Check sheet for the drawn part. Datum: minimum x, y, z corner. Units: mm. A direction names the side the tool comes from. Give positions to 0.01 mm unless a question says otherwise; leave off trailing zeros. Write each loop counter-clockwise with the first axis right and the second up, starting at its lowest first coordinate (ties: lowest second). Pieces come first, ordered by that corner, then holes. Notation, with made-up numbers: (-32.75, 20.5) - (-13.75, 20.5) arc R13 ccw to (-13.75, 26.5) - close; hole circle Ø5 at (10, 27). An arc over 180 degrees is marked (long way). Return JSON: item names as keys, results as strings. Group by question number.
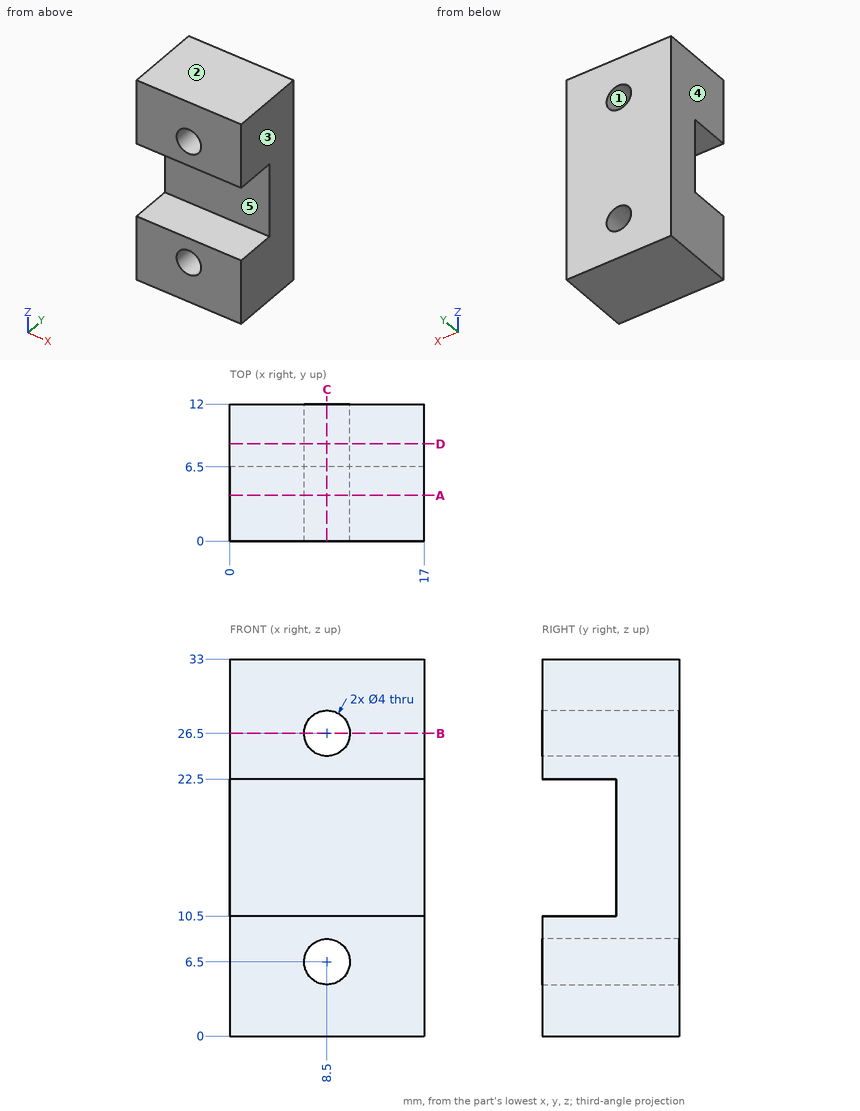
Item 1: Material ranges on line 1 along Z through (x, y) = (1, 2.25); line 2 along X through (y, z) = (5.25, 6.5); line 3 along Z through (x, y) = (6.75, 3.5), recorded low to high. Write a range as from..to.
Item 2: Section check B-B on z = 26.5. Record the cut outline in (x, y), plus the area to 3 significant figures.
Item 3: Access from +Z, -Z, +X, -X, +Y, -Y to the whole of each face (thin tool, end or side, straight path). Record for the marked faces 4 and 5.
Item 4: Mould release check, pull along X, two halves, no side actions. Record for the marked faces 1, 2 and 3: +X half, -X half, draft (parallel to the pull), parting line (faces both ways), or undercut.
Item 5: Section check A-A on y = 4. Record the cut outline in (x, z).
Item 6: Section check D-D on y = 8.5. Record the cut outline in (x, z).
Item 7: Section check C-C on x = 8.5. Record the cut outline in (y, z).
Reply:
{
 "1": {"line 1": "0..10.5, 22.5..33", "line 2": "0..6.5, 10.5..17", "line 3": "0..5.53, 7.47..10.5, 22.5..25.53, 27.47..33"},
 "2": {"outline": "(0, 0) - (6.5, 0) - (6.5, 12) - (0, 12) - close; (10.5, 0) - (17, 0) - (17, 12) - (10.5, 12) - close", "area": "156 mm²"},
 "3": {"face 4": "+Z, -Z, -X, +Y, -Y", "face 5": "+X, -X, -Y"},
 "4": {"face 1": "undercut", "face 2": "draft", "face 3": "+X half"},
 "5": {"outline": "(0, 0) - (17, 0) - (17, 10.5) - (0, 10.5) - close; (0, 22.5) - (17, 22.5) - (17, 33) - (0, 33) - close; hole circle Ø4 at (8.5, 6.5); hole circle Ø4 at (8.5, 26.5)"},
 "6": {"outline": "(0, 0) - (17, 0) - (17, 33) - (0, 33) - close; hole circle Ø4 at (8.5, 6.5); hole circle Ø4 at (8.5, 26.5)"},
 "7": {"outline": "(0, 0) - (12, 0) - (12, 4.5) - (0, 4.5) - close; (0, 8.5) - (12, 8.5) - (12, 24.5) - (0, 24.5) - (0, 22.5) - (6.5, 22.5) - (6.5, 10.5) - (0, 10.5) - close; (0, 28.5) - (12, 28.5) - (12, 33) - (0, 33) - close"}
}
